from build123d import *

# Parameters (mm, degrees)
CROQUIS1_W              = 544
CROQUIS1_H              = 20
SALIENTE_EXTRUIR1_DEPTH = 6
CROQUIS3_W              = 40
CROQUIS3_H              = 6
CORTAR_EXTRUIR1_DEPTH   = 6
MATRIZL1_COUNT          = 7
MATRIZL1_PITCH          = 80
CROQUIS4_W              = 24
CROQUIS4_H              = 6
CORTAR_EXTRUIR2_DEPTH   = 6
CROQUIS5_W              = 6
CROQUIS5_H              = 8
SALIENTE_EXTRUIR3_DEPTH = 6


with BuildPart() as part:
    # Croquis1 → Saliente-Extruir1 (new body)
    with BuildSketch(Plane(origin=(0, 0, 0), x_dir=(1, 0, 0), z_dir=(0, 1, 0))):
        with Locations((272, 10)):
            Rectangle(CROQUIS1_W, CROQUIS1_H)
    extrude(amount=SALIENTE_EXTRUIR1_DEPTH)

    # Croquis3 → Cortar-Extruir1 (cut)
    with BuildSketch(Plane(origin=(0, 0, 0), x_dir=(1, 0, 0), z_dir=(0, 1, 0))):
        with Locations((20, 3)):
            Rectangle(CROQUIS3_W, CROQUIS3_H)
    cortar_extruir1 = extrude(amount=CORTAR_EXTRUIR1_DEPTH, mode=Mode.SUBTRACT)

    # MatrizL1: Cortar-Extruir1 ×7
    with Locations(*[(i * MATRIZL1_PITCH, 0, 0) for i in range(1, MATRIZL1_COUNT)]):
        add(cortar_extruir1, mode=Mode.SUBTRACT)

    # Croquis4 → Cortar-Extruir2 (cut)
    with BuildSketch(Plane(origin=(0, 6, 0), x_dir=(1, 0, 0), z_dir=(0, 1, 0))):
        with Locations((532, 3)):
            Rectangle(CROQUIS4_W, CROQUIS4_H)
    extrude(amount=-CORTAR_EXTRUIR2_DEPTH, mode=Mode.SUBTRACT)

    # Croquis5 → Saliente-Extruir3 (add)
    with BuildSketch(Plane(origin=(0, 0, 0), x_dir=(1, 0, 0), z_dir=(0, 1, 0))):
        with Locations((-3, 10)):
            Rectangle(CROQUIS5_W, CROQUIS5_H)
        with Locations((547, 10)):
            Rectangle(CROQUIS5_W, CROQUIS5_H)
    extrude(amount=SALIENTE_EXTRUIR3_DEPTH)


solid = part.part
Model file for the job. Use its own axes, mm. Coordinates: 2 decimals unless noted, no trailing zeros. Order: outer loops, then holes, each group sorted by start corner. A loop starts at its lowest first (then second) coordinate and runs counter-clockwise, first axis right, second up. Notation, with made-up numbers: M -3,-4.5 L 51,-4.5 A17 ccw 51,26.5 Z; hole C 2.5,24 d5. An arc over 180 degrees is marked long. Return JSON: item names as keys, results as strings.
1. Drill centre lines: probe 1 along X at (y, z) = (0.8, -3.25); probe 2 along X at (y, z) = (3.8, -17); probe 3 along Z at (x, y) = (525, 2.35). Where is each one in solid material? Low to high.
Ans:
{"probe 1": "40 to 80, 120 to 160, 200 to 240, 280 to 320, 360 to 400, 440 to 480", "probe 2": "0 to 544", "probe 3": "-20 to -6"}
2. Flat gauge pins, fed straight in: pin 1 (1.8 mm diameter, centred on x = 250, y = 3.5, fed in from +Z); pin 2 (3 mm diameter, centred on x = -4, y = 3.5, fed in from -Z); pin 3 (3 mm diameter, centred on y = 3.5, z = -2, fed in from +X). Where does each tip first touch, or does it go through?
Ans:
{"pin 1": "z = -6", "pin 2": "z = -14", "pin 3": "x = 480"}
3. Saw through at B-B (x = 416.5). Give the cut face in (y, z).
Ans:
{"outline": "M 0,-20 L 6,-20 L 6,-6 L 0,-6 Z"}
